Can you work these out from the model? Positions are in its coordinate system, mm. A direction names the side the tool comes from. Round coordinates to 2 decimals unless told otherwise and drop trailing zeros. Order: outer loops, then holes, each group sorted by start corner. A loop starts at its lowest first (then second) coordinate and runs counter-clockwise, first axis right, second up.
Q1. If we section it at A-A (z = -101.5): Please give me the cut outline in (x, y), plus the area to 3 significant figures.
Q2. If we section it at B-B (x = 23.5): Please give me the cut outline in (y, z), plus the area to 3 significant figures.
Q3. Will these pins go through, and if not, where does the flat tip stop? P1, Ø3, axis at x = -192, z = 8, coming from the -Y side; P2, Ø6, axis at x = 169, y = 476.5, coming from the +Z side; P3, Ø1.5, axis at y = -45, z = 415.5, coming from the +X side.
Q4. If we section it at D-D (y = 667.5): Please give me the cut outline in (x, z).
Q5. If I drill on line 1 (Y direction, x = -63.5, z = 159); line 2 (Y direction, x = -110, z = 58); line 3 (Z direction, x = 76.5, y = 139.5), over which ranges is the centre line in solid material (lowest first)?
Q6. For faces 1 (the face through (-3, -520, 609)), 2 (the face through (197, 570, -47)), 3 (the face through (-195, 570, -43)), 4 (the face through (-3, -372, 340)), 5 (the face through (210, -73, 316)), which set-ups out of +Z, -Z, +X, -X, +Y, -Y let a thin tool reach every point of the face, with its end or its side?
Q7. If we section it at C-C (y = -188.5): Please give me the cut outline in (x, z), plus the area to 3 significant figures.
from build123d import *

# Parameters (mm, degrees)
BOSS_EXTRUDE1_DEPTH = 210
SKETCH3_W           = 270
SKETCH3_H           = 330
BOSS_EXTRUDE2_DEPTH = 320
SKETCH4_W           = 330
SKETCH4_H           = 425
BOSS_EXTRUDE3_DEPTH = 257.5
SKETCH5_W           = 420
SKETCH5_H           = 220
BOSS_EXTRUDE4_DEPTH = 490
SKETCH6_W           = 420
SKETCH6_H           = 100
BOSS_EXTRUDE5_DEPTH = 100


with BuildPart() as part:
    # Sketch2 → Boss-Extrude1 (new, symmetric)
    with BuildSketch(Plane(origin=(0, 0, 0), x_dir=(0, 0, -1), z_dir=(1, 0, 0))):
        Polygon((-560, -130), (210, -130), (210, 570), (-120, 570), (-120, 45), (-560, 45), align=None)
    extrude(amount=BOSS_EXTRUDE1_DEPTH, both=True)

    # Sketch3 → Boss-Extrude2 (add)
    with BuildSketch(Plane(origin=(0, 570, 0), x_dir=(1, 0, 0), z_dir=(0, 1, 0))):
        with Locations((0, 45)):
            Rectangle(SKETCH3_W, SKETCH3_H)
    extrude(amount=BOSS_EXTRUDE2_DEPTH)

    # Sketch4 → Boss-Extrude3 (add, symmetric)
    with BuildSketch(Plane(origin=(0, 0, 0), x_dir=(0, 0, -1), z_dir=(1, 0, 0))):
        with Locations((45, 357.5)):
            Rectangle(SKETCH4_W, SKETCH4_H)
    extrude(amount=BOSS_EXTRUDE3_DEPTH, both=True)

    # Sketch5 → Boss-Extrude4 (add)
    with BuildSketch(Plane.XZ.offset(130)):
        with Locations((0, 450)):
            Rectangle(SKETCH5_W, SKETCH5_H)
    extrude(amount=BOSS_EXTRUDE4_DEPTH)

    # Sketch6 → Boss-Extrude5 (add)
    with BuildSketch(Plane.XY.offset(560)):
        with Locations((0, -570)):
            Rectangle(SKETCH6_W, SKETCH6_H)
    extrude(amount=BOSS_EXTRUDE5_DEPTH)


solid = part.part
Solution:
1. outline: (-257.5, 145) - (-210, 145) - (-210, -130) - (210, -130) - (210, 145) - (257.5, 145) - (257.5, 570) - (135, 570) - (135, 890) - (-135, 890) - (-135, 570) - (-257.5, 570) - close
1. area: 421,000 mm2
2. outline: (-620, 340) - (-130, 340) - (-130, -210) - (890, -210) - (890, 120) - (45, 120) - (45, 560) - (-520, 560) - (-520, 660) - (-620, 660) - close
2. area: 531,000 mm2
3. P1: stops at y = -130
3. P2: stops at z = 120
3. P3: stops at x = 210
4. outline: (-135, -210) - (135, -210) - (135, 120) - (-135, 120) - close
5. line 1: y = -130 to 45
5. line 2: y = -130 to 890
5. line 3: z = -210 to 120
6. face 1: +Z, +X, -X, +Y
6. face 2: +Z, -Z, +X, +Y
6. face 3: +Z, -Z, -X, +Y
6. face 4: -Z, +X, -X, -Y
6. face 5: +Z, -Z, +X, -Y
7. outline: (-210, 340) - (210, 340) - (210, 560) - (-210, 560) - close
7. area: 92,400 mm2
